from build123d import *

# Parameters (mm, degrees)
SKETCH1_W           = 29.972
SKETCH1_H           = 10.668
BOSS_EXTRUDE1_DEPTH = 1.651
SKETCH2_W           = 4.191
SKETCH2_H           = 5.08
BOSS_EXTRUDE2_DEPTH = 0.889
SKETCH3_R           = 0.381
CUT_EXTRUDE1_DEPTH  = 32.856754527


with BuildPart() as part:
    # Sketch1 → Boss-Extrude1 (new body)
    with BuildSketch(Plane(origin=(0, 0, 0), x_dir=(1, 0, 0), z_dir=(0, 1, 0))):
        with Locations((14.986, 5.334)):
            Rectangle(SKETCH1_W, SKETCH1_H)
    extrude(amount=BOSS_EXTRUDE1_DEPTH)

    # Sketch2 → Boss-Extrude2 (add)
    with BuildSketch(Plane(origin=(0, 1.651, 0), x_dir=(1, 0, 0), z_dir=(0, 1, 0))):
        with Locations((14.986, 5.334)):
            Rectangle(SKETCH2_W, SKETCH2_H)
        with Locations((9.017, 5.334)):
            Rectangle(SKETCH2_W, SKETCH2_H)
        with Locations((20.955, 5.334)):
            Rectangle(SKETCH2_W, SKETCH2_H)
    extrude(amount=BOSS_EXTRUDE2_DEPTH)

    # Sketch3 → Cut-Extrude1 (cut, through all)
    with BuildSketch(Plane(origin=(0, 1.651, 0), x_dir=(1, 0, 0), z_dir=(0, 1, 0))):
        with Locations(Location((26.797, 1.524, 0), (0, 0, 270))):
            Circle(SKETCH3_R)
        with Locations(Location((26.797, 4.064, 0), (0, 0, 270))):
            Circle(SKETCH3_R)
        with Locations(Location((26.797, 6.604, 0), (0, 0, 90))):
            Circle(SKETCH3_R)
        with Locations(Location((26.797, 9.144, 0), (0, 0, 90))):
            Circle(SKETCH3_R)
        with Locations(Location((3.175, 1.524, 0), (0, 0, 90))):
            Circle(SKETCH3_R)
        with Locations(Location((3.175, 4.064, 0), (0, 0, 90))):
            Circle(SKETCH3_R)
        with Locations(Location((3.175, 6.604, 0), (0, 0, 270))):
            Circle(SKETCH3_R)
        with Locations(Location((3.175, 9.144, 0), (0, 0, 270))):
            Circle(SKETCH3_R)
    extrude(amount=-CUT_EXTRUDE1_DEPTH, mode=Mode.SUBTRACT)


solid = part.part
Verification items for the finished model (mm, model axes). A direction names the side the tool comes from. Give positions to 0.01 mm unless a question says otherwise; leave off trailing zeros. Loops run counter-clockwise (first coordinate to the right, second up) from the corner with the lowest first, then second, coordinate; pieces in that order, holes last. Notation, with made-up numbers: (-7, -12.5) - (26, -12.5) arc R14 ccw to (26, -7.5) - close; hole circle Ø7 at (63, 88.5). An arc over 180 degrees is marked (long way). Write item = value, one per line. Start each with the question number.
Q1. Mould release check, pull along Z, two halves, no side actions. Record for faces 5 (the face through (18.859, 2, -5)), 6 (the face through (21, 2, -2.794)), 7 (the face through (15, 1, -10.668)): released by +Z, released by -Z, zero draft, split by the parting line, or undercut.
Q2. Cross-section at A-A, the plane z = -1.5. Enter the section's corners in (x, y).
Q3. Cross-section at C-C, the plane z = -4.75. Enter the section's corners in (x, y), and give its area (3 significant figures).
Q4. Tool access check on faces 1 (the face through (12.891, 2, -5)), 2 (the face through (6.922, 2, -5)), 3 (the face through (15, 2, -2.794)), 4 (the face through (21, 2, -7.874)). Record the directions out of +Z, -Z, +X, -X, +Y, -Y that give a thin tool (end or side, any length) a straight path to the whole face; none if there is none.
Q5. Thickness scan on line 1 (X direction, y = 1.7, z = -4.5); line 2 (Z direction, x = 8.5, y = 2.35); line 3 (Y direction, x = 19, z = -2.25). Record the ranges inside material, lowest first.
Q6. Depth check by flat-ended pin: P1, Ø1, axis at y = 2, z = -4, coming from the -X side; P2, Ø1, axis at y = 2.5, z = -5.5, coming from the +X side; P3, Ø1.5, axis at x = 27, z = -4.5, coming from the +Y side. Enter the tip coordinate at first touch or a pass-through.
Q7. Cross-section at B-B, the plane x = 7.5. Enter the section's corners in (y, z), and give its area (3 significant figures).
Q8. Cross-section at D-D, the plane x = 24.5. Enter the section's corners in (y, z).
Answer key:
q1.face_5 = zero draft
q1.face_6 = released by +Z
q1.face_7 = released by -Z
q2.outline = (0, 0) - (2.79, 0) - (2.79, 1.65) - (0, 1.65) - close; (3.56, 0) - (26.42, 0) - (26.42, 1.65) - (3.56, 1.65) - close; (27.18, 0) - (29.97, 0) - (29.97, 1.65) - (27.18, 1.65) - close
q3.outline = (0, 0) - (29.97, 0) - (29.97, 1.65) - (23.05, 1.65) - (23.05, 2.54) - (18.86, 2.54) - (18.86, 1.65) - (17.08, 1.65) - (17.08, 2.54) - (12.89, 2.54) - (12.89, 1.65) - (11.11, 1.65) - (11.11, 2.54) - (6.92, 2.54) - (6.92, 1.65) - (0, 1.65) - close
q3.area = 60.7 mm^2
q4.face_1 = +Z, -Z, +Y
q4.face_2 = +Z, -Z, -X, +Y
q4.face_3 = +Z, +X, -X, +Y
q4.face_4 = -Z, +X, -X, +Y
q5.line_1 = 6.92 to 11.11, 12.89 to 17.08, 18.86 to 23.05
q5.line_2 = -7.87 to -2.79
q5.line_3 = 0 to 1.65
q6.P1 = 0
q6.P2 = 23.05
q6.P3 = 1.65
q7.outline = (0, -10.67) - (1.65, -10.67) - (1.65, -7.87) - (2.54, -7.87) - (2.54, -2.79) - (1.65, -2.79) - (1.65, 0) - (0, 0) - close
q7.area = 22.1 mm^2
q8.outline = (0, -10.67) - (1.65, -10.67) - (1.65, 0) - (0, 0) - close
